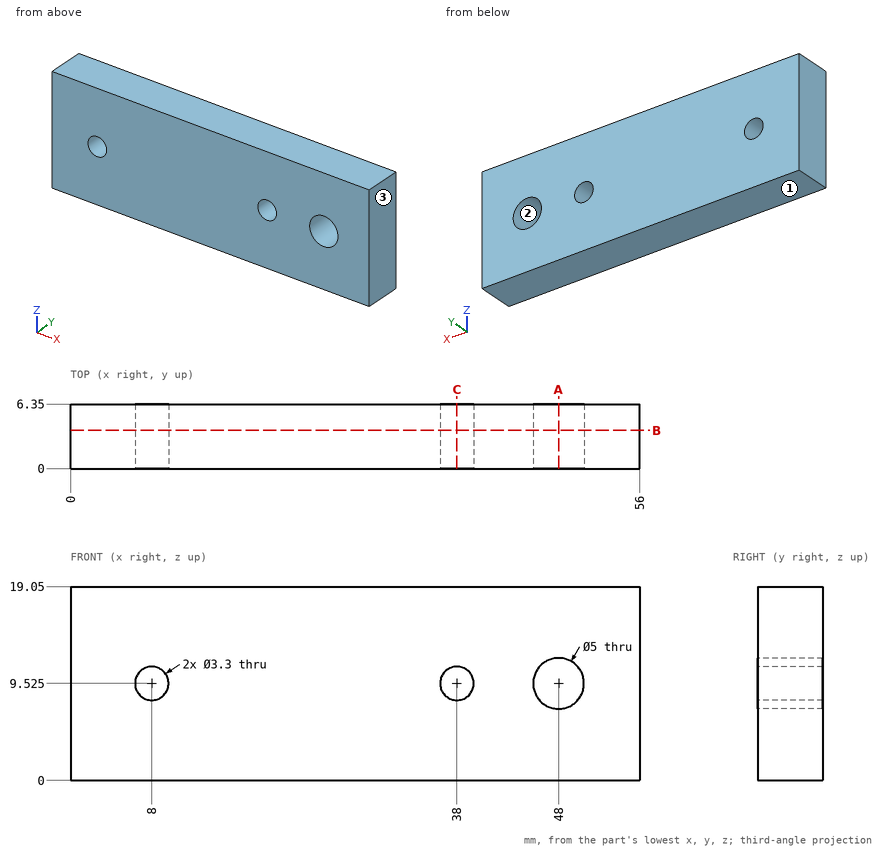
Geometry: see drawing. Coordinates: mm, zero at the bounding-box minimum. Coordinates: 2 decimals unless noted, no trailing zeros. Loops run counter-clockwise (first coordinate to the right, second up) from the corner with the lowest first, then second, coordinate; pieces in that order, holes last.
(1) Pull-direction query (Z, two-part tool) for the marked faces 1, 2 and 3; classes: released by +Z, released by -Z, zero draft, split by the parting line, or undercut.
(2) Section C-C on x = 38. Return the cut outline in (y, z) (3 decimals).
(3) Material intervals for probe 1 along X at (y, z) = (1.5, 10); probe 2 along X at (y, z) = (1.75, 11); probe 3 along Z at (x, y) = (9, 3.25), sorted ascending.
(4) Section A-A on x = 48. Return the cut outline in (y, z) (3 decimals).
(5) Section B-B on y = 3.75. Return the cut outline in (x, z) (3 decimals), then the cut area to 3 significant figures.
Data:
1. face 1: released by -Z
1. face 2: undercut
1. face 3: zero draft
2. outline: (0, 0) - (6.35, 0) - (6.35, 7.875) - (0, 7.875) - close; (0, 11.175) - (6.35, 11.175) - (6.35, 19.05) - (0, 19.05) - close
3. probe 1: x = 0 to 6.42, 9.58 to 36.42, 39.58 to 45.55, 50.45 to 56
3. probe 2: x = 0 to 7.26, 8.74 to 37.26, 38.74 to 45.98, 50.02 to 56
3. probe 3: z = 0 to 8.21, 10.84 to 19.05
4. outline: (0, 0) - (6.35, 0) - (6.35, 7.025) - (0, 7.025) - close; (0, 12.025) - (6.35, 12.025) - (6.35, 19.05) - (0, 19.05) - close
5. outline: (0, 0) - (56, 0) - (56, 19.05) - (0, 19.05) - close; hole circle Ø3.3 at (8, 9.525); hole circle Ø3.3 at (38, 9.525); hole circle Ø5 at (48, 9.525)
5. area: 1,030 mm2
